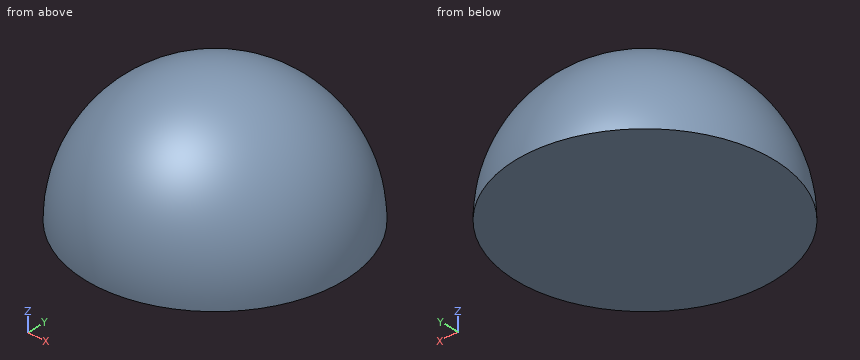
```python
from build123d import *

# Parameters (mm, degrees)
F2_W     = 29.3561853468
F2_H     = 76.5563324094
F3_DEPTH = 50.8
F4_W     = 76.2685239315
F4_H     = 38.5659746826
F5_DEPTH = 25.4


with BuildPart() as f1:
    # F0 (on Top) → F1 (revolve)
    with BuildSketch(Plane.XY):
        with BuildLine():
            Line((0, 19.05), (0, -19.05))
            ThreePointArc((0, -19.05), (19.05, 0), (0, 19.05))
        make_face()
    revolve(axis=Axis((0, 0, 0), (0, -1, 0)))

    # F2 (on Top) → F3 (cut)
    with BuildSketch(Plane.XY):
        with Locations((14.6780926734, -3.4536682069)):
            Rectangle(F2_W, F2_H)
    extrude(amount=-F3_DEPTH, mode=Mode.SUBTRACT)

    # F4 (on Right) → F5 (cut)
    with BuildSketch(Plane.YZ):
        with Locations((3.5975724459, -19.2829873413)):
            Rectangle(F4_W, F4_H)
    extrude(amount=-F5_DEPTH, mode=Mode.SUBTRACT)


solid = f1.part
```
Source: CAD feature listing. Evaluate the final solid. Frame: model axes, mm. Coordinates: 2 decimals unless noted, no trailing zeros. Write each loop counter-clockwise with the first axis right and the second up, starting at its lowest first coordinate (ties: lowest second). Pieces come first, ordered by that corner, then holes. Notation, with made-up numbers: (-18.5, -38) - (26.5, -38) arc R28 cw to (26.5, -5) - close; hole circle Ø7 at (80, 53.5). An arc over 180 degrees is marked (long way). Answer as a JSON object with one key per item and string values.
Q1. First-contact query: pin 1 Ø6 at (y, z) = (-9.5, 16) entering from -X; pin 2 Ø4 at (x, y) = (9.5, 0.5) entering from -Z; pin 3 Ø12 at (x, y) = (7, -8) entering from +Z; pin 4 Ø2 at (x, z) = (-11, 5) entering from -Y. Flat tips, straight axial feed; report the tip coordinate or a pass-through.
Ans:
{"pin 1": "stops at x = -10.92", "pin 2": "stops at z = 0", "pin 3": "stops at z = 18.48", "pin 4": "stops at y = -15.49"}
Q2. Material intervals for line 1 (Z direction, x = -12, y = 10.5); line 2 (X direction, y = -17, z = 4.5); line 3 (Y direction, x = -3.5, z = 2), sorted ascending. Write a range as [from, to].
Ans:
{"line 1": "z = [0, 10.42]", "line 2": "x = [-7.32, 7.32]", "line 3": "y = [-18.62, 18.62]"}
Q3. Section query C-C, the plane z = 8. Output: boundary loops of the cut face in (x, y).
Ans:
{"outline": "circle Ø34.58 at (0, 0)"}
Q4. Section query D-D, the plane z = 15.75. Output: boundary loops of the cut face in (x, y), plus the area to 3 significant figures.
Ans:
{"outline": "circle Ø21.43 at (0, 0)", "area": "361 mm2"}
Q5. Section query A-A, the plane y = -9. Output: boundary loops of the cut face in (x, z), plus the area to 3 significant figures.
Ans:
{"outline": "(-16.79, 0) - (16.79, 0) arc R16.79 ccw to start", "area": "443 mm2"}
Q6. Section query B-B, the plane x = -9.5. Output: boundary loops of the cut face in (y, z).
Ans:
{"outline": "(-16.51, 0) - (16.51, 0) arc R16.51 ccw to start"}
